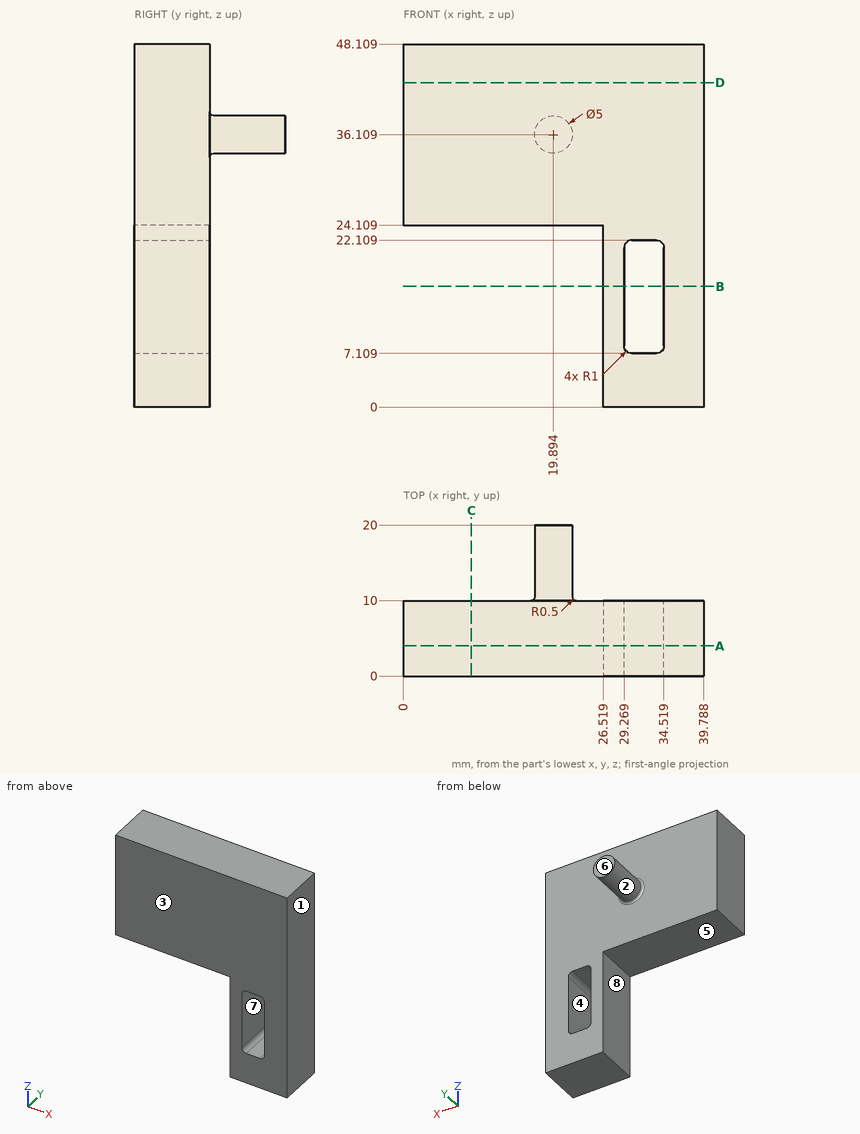
Could you check a few things on this drawing? It's one solid part, dimensions in mm from its lowest x, y, z. A direction names the side the tool comes from. Coordinates: 2 decimals unless noted, no trailing zeros. Write each loop counter-clockwise with the first axis right and the second up, starting at its lowest first coordinate (ties: lowest second). Pieces come first, ordered by that corner, then holes. Notation, with made-up numbers: (36.25, 41.25) - (90.25, 41.25) arc R22 ccw to (90.25, 65.25) - close; hole circle Ø10 at (43, 25.5). An arc over 180 degrees is marked (long way). Put each result on its own line as item: value. Start each with the question number.
Q1. Please list where these lines run through material, in increasing order: L1, parallel to X at y = 1, z = 15; L2, parallel to Y at x = 28.5, z = 3.5; L3, parallel to Z at x = 11.5, y = 8.
Q2. I want a section at A-A on y = 4. Write out the boundary of the cut face in (x, z), plus the area to 3 significant figures.
Q3. Which directions (+Z, -Z, +X, -X, +Y, -Y) give clear straight access to the entire face, cutting with the end or side of a thin tool? Please do the marked faces 1, 2, 3, 4 and 5.
Q4. I want a section at B-B on z = 16. Write out the boundary of the cut face in (x, y).
Q5. I want a section at D-D on z = 43. Write out the boundary of the cut face in (x, y).
Q6. I want a section at C-C on x = 9. Write out the boundary of the cut face in (y, z).
Q7. Thinking about a two-plate mould opening in X: for the marked faces 6, 7 and 8, which applies, pulls with the +X half, pulls with the -X half, needs draft (parallel to the pull), parting line crosses it, or undercut?
Q8. I'm going to push flat-ended pins straight in: P1, Ø1.5, axis at x = 34, z = 31.5, coming from the -Y side; P2, Ø5, axis at x = 14, y = 6.5, coming from the -Z side; P3, Ø3, axis at y = 4, z = 13, coming from the -X side; P4, Ø3, axis at x = 24, z = 21.5, coming from the -Y side. Where does each tip first touch, or does it pass through?
Checks:
1. L1: 26.52 to 29.27, 34.52 to 39.79
1. L2: 0 to 10
1. L3: 24.11 to 48.11
2. outline: (0, 24.11) - (26.52, 24.11) - (26.52, 0) - (39.79, 0) - (39.79, 48.11) - (0, 48.11) - close; hole (29.27, 8.11) arc R1 ccw to (30.27, 7.11) - (33.52, 7.11) arc R1 ccw to (34.52, 8.11) - (34.52, 21.11) arc R1 ccw to (33.52, 22.11) - (30.27, 22.11) arc R1 ccw to (29.27, 21.11) - close
2. area: 1,200 mm²
3. face 1: +Z, -Z, +X, +Y, -Y
3. face 2: +Y
3. face 3: +Z, -Z, +X, -X, -Y
3. face 4: +Y, -Y
3. face 5: -Z, -X, +Y, -Y
4. outline: (26.52, 0) - (29.27, 0) - (29.27, 10) - (26.52, 10) - close; (34.52, 0) - (39.79, 0) - (39.79, 10) - (34.52, 10) - close
5. outline: (0, 0) - (39.79, 0) - (39.79, 10) - (0, 10) - close
6. outline: (0, 24.11) - (10, 24.11) - (10, 48.11) - (0, 48.11) - close
7. face 6: needs draft
7. face 7: undercut
7. face 8: pulls with the -X half
8. P1: y = 0
8. P2: z = 24.11
8. P3: x = 26.52
8. P4: through
